Could you check a few things on this drawing? It's one solid part, dimensions in mm from its lowest x, y, z. A direction names the side the tool comes from. Round coordinates to 2 decimals unless told otherwise and drop trailing zeros. Order: outer loops, then holes, each group sorted by start corner. A loop starts at its lowest first (then second) coordinate and runs counter-clockwise, first axis right, second up. Notation, with made-up numbers: M 1.5,42.5 L 19.5,42.5 A16 cw 19.5,60.5 Z; hole C 45,13 d3. An arc over 180 degrees is marked long. Answer as a JSON object with one key per item and string values. Group by question number.
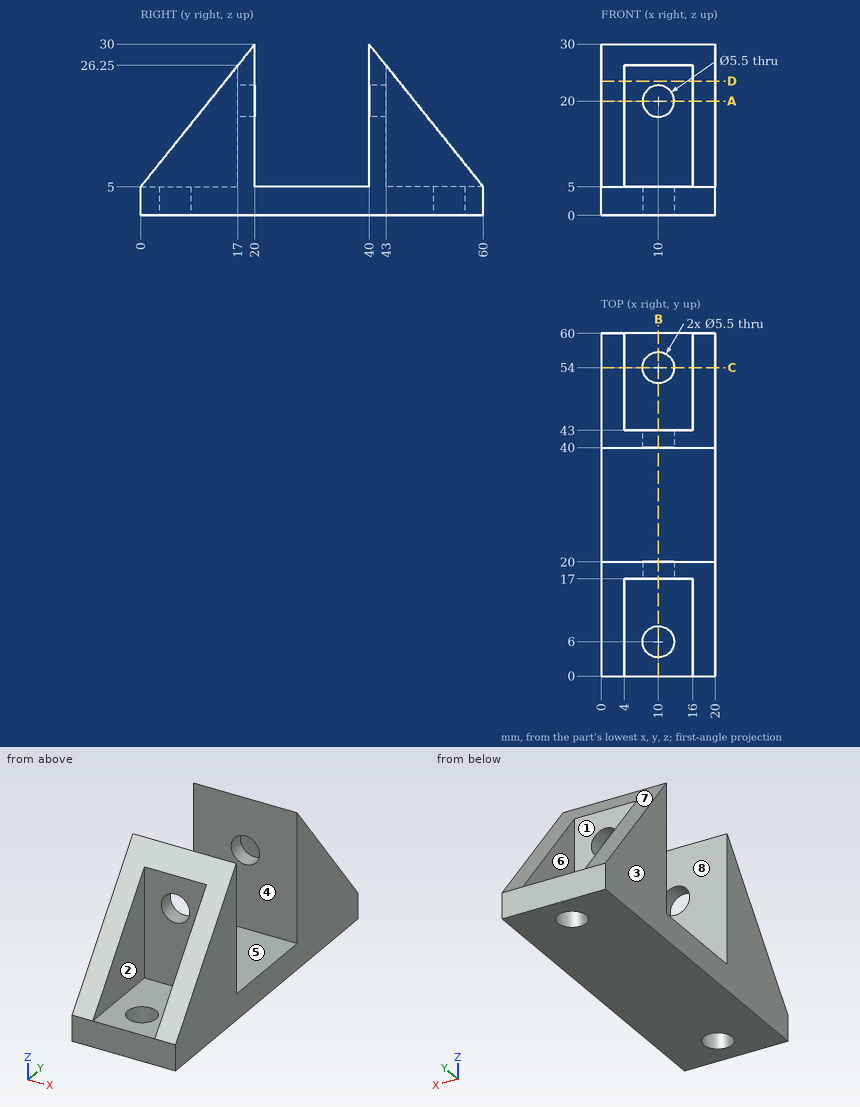
1) We'd pull the mould along Y, two halves only. Please class the marked faces 5, 6, 7 and 8: +Y half, -Y half, draft (parallel to the pull), parting line (faces both ways), or undercut.
2) If we section it at A-A on z = 20: Write out the boundary of the cut face in (x, y).
3) If we section it at B-B on x = 10: Write out the boundary of the cut face in (y, z), plus the area to 3 significant figures.
4) If we section it at C-C on y = 54: Write out the boundary of the cut face in (x, z).
5) Which directions (+Z, -Z, +X, -X, +Y, -Y) give clear straight access to the entire face, cutting with the end or side of a thin tool? Please do the marked faces 1, 2, 3 and 4.
6) For pin 1 (5 mm diameter, centred on x = 10, y = 54, fed in from +Z); pin 2 (3.5 mm diameter, centred on x = 10, z = 15, fed in from -Y); pin 3 (8 mm diameter, centred on x = 11.5, y = 11, fed in from +Z); pin 4 (6 mm diameter, centred on x = 5.5, y = 15.5, fed in from +Z) (3 decimals), each with a flat end and sliding along its axis, tell me the tip position at first contact or that it passes through.
7) If we section it at D-D on z = 23.5: Write out the boundary of the cut face in (x, y).
8) I need wall thicknesses on line 1 along X through (y, z) = (18.05, 20); line 2 along Y through (x, z) = (13.5, 19); line 3 along Y through (x, z) = (10, 1.7). Which ranges of each line are inside material? Lowest first, please.
Findings:
{
 "1": {"face 5": "undercut", "face 6": "draft", "face 7": "+Y half", "face 8": "undercut"},
 "2": {"outline": "M 0,12 L 4,12 L 4,17 L 7.25,17 L 7.25,20 L 0,20 Z; M 0,40 L 7.25,40 L 7.25,43 L 4,43 L 4,48 L 0,48 Z; M 12.75,17 L 16,17 L 16,12 L 20,12 L 20,20 L 12.75,20 Z; M 12.75,40 L 20,40 L 20,48 L 16,48 L 16,43 L 12.75,43 Z"},
 "3": {"outline": "M 0,0 L 3.25,0 L 3.25,5 L 0,5 Z; M 8.75,0 L 51.25,0 L 51.25,5 L 43,5 L 43,17.25 L 40,17.25 L 40,5 L 20,5 L 20,17.25 L 17,17.25 L 17,5 L 8.75,5 Z; M 17,22.75 L 20,22.75 L 20,30 L 17,26.25 Z; M 40,22.75 L 43,22.75 L 43,26.25 L 40,30 Z; M 56.75,0 L 60,0 L 60,5 L 56.75,5 Z", "area": "351 mm^2"},
 "4": {"outline": "M 0,0 L 7.25,0 L 7.25,5 L 4,5 L 4,12.5 L 0,12.5 Z; M 12.75,0 L 20,0 L 20,12.5 L 16,12.5 L 16,5 L 12.75,5 Z"},
 "5": {"face 1": "+Z, +Y", "face 2": "+Z, -Y", "face 3": "+Z, -Z, -X, +Y, -Y", "face 4": "+Z, +X, -X"},
 "6": {"pin 1": "passes through", "pin 2": "stops at y = 17", "pin 3": "stops at z = 5", "pin 4": "stops at z = 28.125"},
 "7": {"outline": "M 0,14.8 L 4,14.8 L 4,17 L 16,17 L 16,14.8 L 20,14.8 L 20,20 L 0,20 Z; M 0,40 L 20,40 L 20,45.2 L 16,45.2 L 16,43 L 4,43 L 4,45.2 L 0,45.2 Z"},
 "8": {"line 1": "x = 0 to 7.25, 12.75 to 20", "line 2": "y = 17 to 20, 40 to 43", "line 3": "y = 0 to 3.25, 8.75 to 51.25, 56.75 to 60"}
}
